The model under review builds one solid part; all positions refer to its coordinate system, in mm. A direction names the side the tool comes from. Give positions to 0.01 mm unless a question says otherwise; leave off trailing zeros. Order: outer loops, then holes, each group sorted by start corner. A loop starts at its lowest first (then second) coordinate and runs counter-clockwise, first axis right, second up.
Autodesk Inventor part; units mm, degrees
ref_plane "YZ Plane" through (0, 0, 0) normal (1, 0, 0) x (0, 1, 0)
ref_plane "XZ Plane" through (0, 0, 0) normal (0, 1, 0) x (-1, 0, 0)
ref_plane "XY Plane" through (0, 0, 0) normal (0, 0, 1) x (1, 0, 0)
ref_plane "工作平面1" through (19.3371, -7.6679, 114.989) normal (-1, 0, 0) x (0, -1, 0)
sketch "草图1" plane through (19.3371, -7.6679, 114.989) normal (-1, 0, 0) x (0, -1, 0)
  circle A0 centre (20, 75) radius 2.1
  circle A1 centre (20, 90) radius 2.1
  circle A2 centre (20, 60) radius 2.1
  circle A3 centre (8, 60) radius 2.1
  circle A4 centre (8, 90) radius 2.1
  line L0 (0, 0) -> (0, 214)
  circle A5 centre (12.0096, 5) radius 2.1
  circle A6 centre (25, 12.5) radius 2.1
  circle A7 centre (37.9904, 5) radius 2.1
  circle A8 centre (20, 75) radius 2.1
  circle A9 centre (20, 90) radius 2.1
  circle A10 centre (20, 60) radius 2.1
  circle A11 centre (8, 90) radius 2.1
  circle A12 centre (8, 60) radius 2.1
  circle A13 centre (15.7729, 200.5) radius 2.1
  circle A14 centre (28.7632, 208) radius 2.1
  circle A15 centre (28.7632, 178) radius 2.1
  circle A16 centre (15.7729, 185.5) radius 2.1
  circle A17 centre (41.7536, 200.5) radius 2.1
  circle A18 centre (41.7536, 185.5) radius 2.1
  circle A19 centre (28.7632, 193) radius 7.5
  arc A20 (48.2862, 199.5655) -> (25.6285, 214) centre (25.6285, 189) ccw
  line L1 (25.6285, 214) -> (0, 214)
  line L2 (0, 0) -> (0, 214)
  line L3 (0, 0) -> (64, 0)
  line L4 (64, 0) -> (64, 23)
  line L5 (66.8284, 25) -> (64, 23)
  line L6 (66.8284, 25) -> (70, 25)
  line L7 (70, 25) -> (70, 147.4576)
  arc A21 (70, 147.4576) -> (67.6577, 158.0231) centre (45, 147.4576) ccw
  line L8 (67.6577, 158.0231) -> (48.2862, 199.5655)
  circle A22 centre (64.4234, 100.25) radius 2.1
  circle A23 centre (37.5766, 49.75) radius 2.1
  circle A24 centre (64.4234, 65.25) radius 2.1
  circle A25 centre (37.5766, 100.25) radius 2.1
  circle A26 centre (64.4234, 84.75) radius 2.1
  circle A27 centre (51, 42) radius 2.1
  circle A28 centre (64.4234, 49.75) radius 2.1
  circle A29 centre (51, 108) radius 2.1
  circle A30 centre (33.7425, 67) radius 3.25
  circle A31 centre (59, 75) radius 3.25
  circle A32 centre (33.7425, 83) radius 3.25
  circle A33 centre (50, 75) radius 3.25
  circle A34 centre (41, 75) radius 3.25
  line L9 (0, 47.65) -> (28, 47.65)
  line L10 (28, 47.65) -> (28, 102.35)
  line L11 (28, 102.35) -> (0, 102.35)
  line L12 (0, 102.35) -> (0, 47.65)
  point P0 (-7.6679, -114.989)
  point P1 (0, 102.35)
  point P2 (0, 47.65)
extrude "拉伸1" add sketch "草图1" along normal blind 7 contours L0 L11 L10 L9
sketch "草图2" plane through (19.3371, -35.6679, 217.339) normal (0, 0, 1) x (1, 0, 0)
  line L0 (-6, -42) -> (-116, -42)
  line L1 (-6, -42) -> (-43, -42)
  line L2 (-43, -42) -> (-43, -14)
  line L3 (-43, -14) -> (-6, -14)
  line L4 (-6, -14) -> (-6, -42)
  line L5 (-48, -3.4068) -> (-48, -11.4068)
  line L6 (-47, -3.4068) -> (-47, 27)
  line L7 (0, 0) -> (-7, 0)
  line L8 (-7, 0) -> (-47, -3.4068)
  line L9 (-47, -3.4068) -> (-47, -42)
  line L10 (0, 0) -> (0, -3)
  line L11 (0, -3) -> (-44, -6.7475)
  line L12 (-44, -6.7475) -> (-44, -42)
  point P0 (-19.3371, 35.6679)
  dimension "d3" = 37
  dimension "d4" = 28
  dimension "d5" = 3
  dimension "d6" = 3
extrude "拉伸2" add sketch "草图2" against normal up to surface (54.7 mm away) contours L0 L9 L8 L7 L10 L11 L12
chamfer "倒角1" distance 2 angle 45 1 edges at (-24.6629, -42.4154, 189.989)
sketch "草图3" plane through (-24.6629, -77.6679, 217.339) normal (1, 0, 0) x (0, 0, -1)
  line L0 (0, 0) -> (0, 33.2525)
  line L1 (0, 0) -> (80, 0)
  line L2 (80, 0) -> (80, 4)
  line L3 (80, 4) -> (0, 4)
  line L4 (0, 4) -> (0, 0)
  point P0 (217.339, 77.6679)
  point P1 (0, 4)
  dimension "d12" = 80
  dimension "d13" = 4
extrude "拉伸3" add sketch "草图3" along normal blind 35
chamfer "倒角2" distance 2 angle 45 8 edges at (10.3371, -75.6679, 217.339) (10.3371, -75.6679, 137.339) (-27.6629, -39.0748, 189.989) (-24.6629, -75.6679, 137.339) (-24.6629, -75.6679, 162.639) (12.3371, -35.6679, 189.989) (19.3371, -38.6679, 189.989) (-27.6629, -77.6679, 189.989)
sketch "草图4" plane through (-24.6629, -73.6679, 217.339) normal (0, 1, 0) x (1, 0, 0)
  line L0 (2, 80) -> (33, 80)
  line L1 (19, 80) -> (19, -0.4467) construction
  line L2 (0, 78) -> (0, 56.7)
  line L3 (44, -44.0038) -> (44, 260.8962)
  circle A0 centre (19, 69) radius 1.9
  circle A1 centre (19, 7) radius 1.9
  point P0 (24.6629, 217.339)
  dimension "d19" = 19
  dimension "d20" = 25
  dimension "d21" = 3.8
  dimension "d22" = 3.8
  dimension "d23" = 62
  dimension "d24" = 11
extrude "拉伸4" cut sketch "草图4" against normal blind 35
properties part number "电气支架_2"
Item 1: Take a section at B-B (z = 186.5). Give the boundary of the cut face in (x, y), and give its area (3 significant figures).
Values found:
outline: (-27.66, -75.67) - (-25.66, -77.67) - (10.34, -77.67) - (10.34, -73.67) - (-24.66, -73.67) - (-24.66, -44.42) - (-22.67, -42.25) - (17.34, -38.84) - (19.34, -36.67) - (19.34, -7.67) - (12.34, -7.67) - (12.34, -33.67) - (10.34, -35.84) - (-25.67, -38.9) - (-27.66, -41.07) - close
area: 606 mm2
Item 2: For faces 4 (the flat face through (-23.68, -43.346, 190.372)), 5 (the flat face through (-24.663, -76, 150)), 6 (the flat face through (12.337, -20, 190)), list the 3-axis set-ups (+Z, -Z, +X, -X, +Y, -Y) from which the entire face can be reached by the end or side of a thin tool; tool diameter is ignored.
Values found:
face 4: +Z, -Z, +X
face 5: -Z, -X, +Y, -Y
face 6: +Z, -Z, -X, +Y
Item 3: Take a section at D-D (x = -15.5). Give the boundary of the cut face in (y, z) (3 decimals).
Values found:
outline: (-77.668, 137.339) - (-73.668, 137.339) - (-73.668, 217.339) - (-77.668, 217.339) - close; (-41.635, 162.639) - (-38.039, 162.639) - (-38.039, 217.339) - (-41.635, 217.339) - close
Item 4: For line 1 (Z direction, x = 14.5, y = -25.5); line 2 (X direction, y = -59, z = 164.5); line 3 (X direction, y = -17.5, z = 163.5), list the stretches that pass through material, from the lowest coordinate up.
Values found:
line 1: z = 162.64 to 217.34
line 2: x = -27.66 to -24.66
line 3: x = 12.34 to 19.34
Item 5: Take a section at C-C (y = -15). Give the boundary of the cut face in (x, z).
Values found:
outline: (12.34, 162.64) - (19.34, 162.64) - (19.34, 173) - (12.34, 173) - close; (12.34, 176.98) - (19.34, 176.98) - (19.34, 203) - (12.34, 203) - close; (12.34, 206.98) - (19.34, 206.98) - (19.34, 217.34) - (12.34, 217.34) - close
Item 6: Take a section at A-A (x = -6). Give the boundary of the cut face in (y, z).
Values found:
outline: (-77.67, 137.34) - (-73.67, 137.34) - (-73.67, 146.47) - (-77.67, 146.47) - close; (-77.67, 150.21) - (-73.67, 150.21) - (-73.67, 208.47) - (-77.67, 208.47) - close; (-77.67, 212.21) - (-73.67, 212.21) - (-73.67, 217.34) - (-77.67, 217.34) - close; (-40.83, 162.64) - (-37.23, 162.64) - (-37.23, 217.34) - (-40.83, 217.34) - close
Item 7: Clearance check with flat-ended pins moving along their axes: pin 1 Ø4.5 at (y, z) = (-75.5, 176) entering from +X; pin 2 Ø3 at (x, z) = (-5.66, 210.34) entering from -Y; pin 3 Ø21 at (y, z) = (-16, 198.5) entering from -X. State where each tip first meets the part, or that it passes through.
Values found:
pin 1: stops at x = 10.34
pin 2: stops at y = -40.92
pin 3: stops at x = 12.34
Item 8: Draft analysis for pull direction Y (two halves, no side actions). For faces 1 (the flat face through (-25.677, -75.696, 161.653)), 2 (the flat face through (-26.65, -76.68, 189.1)), 3 (the flat face through (-8, -73.668, 177)), state which applies: released by +Y, released by -Y, zero draft, split by the parting line, or undercut.
Values found:
face 1: zero draft
face 2: released by -Y
face 3: undercut
